The listing builds one solid part. Answer for the finished solid, in the listing's coordinates (mm). Face numbers are marked on the shaded views. A direction names the side the tool comes from. Coordinates: 2 decimals unless noted, no trailing zeros. Loops run counter-clockwise (first coordinate to the right, second up) from the corner with the lowest first, then second, coordinate; pieces in that order, holes last. Notation, with made-up numbers: (1.5, 57.25) - (60.5, 57.25) arc R20 ccw to (60.5, 82.25) - close; hole circle Ø2 at (82.25, 80). An arc over 180 degrees is marked (long way). One line per question, with ' | ' between items.
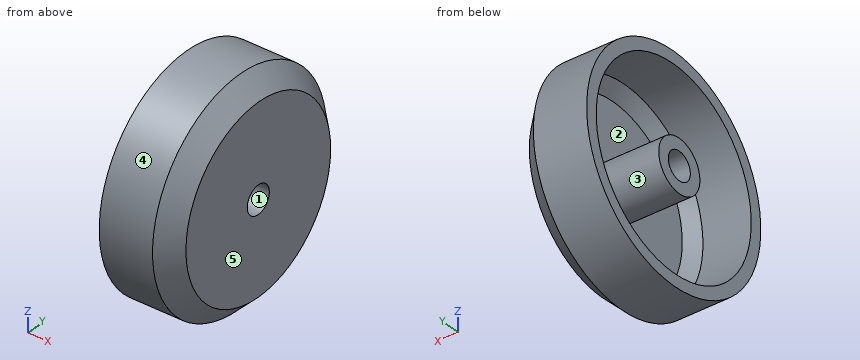
from build123d import *

# Parameters (mm, degrees)
F2_R     = 1.905
F3_DEPTH = 10.542


# Not quite as in the source:
# - a feature names something its author has since deleted; it is built from what else it names


with BuildPart() as f1:
    # F0 (on Front) → F1 (revolve)
    with BuildSketch(Plane.XZ):
        Polygon((8.001, 15.0495), (0.762, 15.0495), (0.762, 13.3985), (7.3171334085, 13.3985), (8.89, 11.8256334085), (8.89, 3.556), (0, 3.556), (0, 0), (10.541, 0), (10.541, 12.5095), align=None)
    revolve(axis=Axis((5.2705, 0, 0), (-1, 0, 0)))

    # F2 (on face) → F3 (cut, through all)
    with BuildSketch(Plane.YZ.offset(10.541)):
        Circle(F2_R)
    extrude(amount=-F3_DEPTH, mode=Mode.SUBTRACT)


solid = f1.part
Item 1: Find section C-C, the plane x = 3.25. Write down the section's boundary in (y, z) (1 decimal).
Taken from the geometry:
outline: circle Ø30.1 at (0, 0); circle Ø7.1 at (0, 0); hole circle Ø26.8 at (0, 0); hole circle Ø3.8 at (0, 0)
Item 2: Each of these flat-tipped pins is pushed along its axis until it touches: pin 1 Ø2 at (x, z) = (8, -10.5) entering from +Y; pin 2 Ø1 at (y, z) = (4.5, 0) entering from -X. Where does it stop, or does it pass through?
Taken from the geometry:
pin 1: stops at y = 11.67 | pin 2: stops at x = 8.89
Item 3: Find the intervals of material crossed by line 1 (X direction, y = 4.5, z = -5); line 2 (Z direction, x = 3.25, y = -1.5); line 3 (Y direction, x = 5.25, z = -10), in increasing order. Write a range as [from, to].
Taken from the geometry:
line 1: x = [8.89, 10.54] | line 2: z = [-14.97, -13.31], [-3.22, -1.17], [1.17, 3.22], [13.31, 14.97] | line 3: y = [-11.25, -8.92], [8.92, 11.25]
Item 4: Which of the six approach directions +Z, -Z, +X, -X, +Y, -Y give full straight-line access (tool end or side, diameter ignored) to the marked faces 1 and 2?
Taken from the geometry:
face 1: +X, -X | face 2: -X
Item 5: Find section A-A, the plane y = 0. Write down the section's boundary in (x, z) (1 decimal), plus the area to 3 significant figures.
Taken from the geometry:
outline: (0, -3.6) - (8.9, -3.6) - (8.9, -11.8) - (7.3, -13.4) - (0.8, -13.4) - (0.8, -15) - (8, -15) - (10.5, -12.5) - (10.5, -1.9) - (0, -1.9) - close; (0, 1.9) - (10.5, 1.9) - (10.5, 12.5) - (8, 15) - (0.8, 15) - (0.8, 13.4) - (7.3, 13.4) - (8.9, 11.8) - (8.9, 3.6) - (0, 3.6) - close | area: 95.6 mm2
Item 6: The mould has two halves that part along Z. Classify the marked faces 3, 4 and 5: pulls with the +Z half, pulls with the -Z half, needs draft (parallel to the pull), parting line crosses it, or undercut.
Taken from the geometry:
face 3: undercut | face 4: parting line crosses it | face 5: needs draft
